Work out the finished part from the listing and answer in its coordinate system (mm). Coordinates: 2 decimals unless noted, no trailing zeros. Order: outer loops, then holes, each group sorted by start corner. A loop starts at its lowest first (then second) coordinate and runs counter-clockwise, first axis right, second up. Notation, with made-up numbers: M 3,7 L 10,7 A22 cw 10,23 Z; hole C 88.5,83 d10. An arc over 180 degrees is marked long. Use a Markdown table: item, result. Add a question column.
from build123d import *

# Parameters (mm, degrees)
SKETCH1_R           = 1.5
BOSS_EXTRUDE1_DEPTH = 40


with BuildPart() as part:
    # Sketch1 → Boss-Extrude1 (new body)
    with BuildSketch(Plane(origin=(0, 0, 0), x_dir=(1, 0, 0), z_dir=(0, 1, 0))):
        Polygon((0, 2.886751346), (-2.5, 1.443375673), (-2.5, -1.443375673), (0, -2.886751346), (2.5, -1.443375673), (2.5, 1.443375673), align=None)
        with Locations(Location((0, 0, 0), (0, 0, 270))):
            Circle(SKETCH1_R, mode=Mode.SUBTRACT)
    extrude(amount=BOSS_EXTRUDE1_DEPTH)

    # Sketch6 → Cut-Revolve1 (revolve, cut)
    with BuildSketch(Plane.ZY):
        Polygon((2.5, 40), (2.886751346, 40), (2.886751346, 39.859234022), align=None)
    cut_revolve1 = revolve(axis=Axis((0, 40, 0), (0, 1, 0)), mode=Mode.SUBTRACT)

    # Mirror1: Cut-Revolve1 across plane
    add(cut_revolve1.mirror(Plane.ZX.offset(20)), mode=Mode.SUBTRACT)


solid = part.part
(1) Given P1, Ø3, axis at x = 1, y = 6.5, coming from the +Z side, flat-ended and moving along its own axis, determine where the tip first touches the part or whether it passes through.
(2) The mould has two halves that part along X. Classify faces 1 (the flat face through (-2.5, 20, 0)), 2 (the conical face through (2.31, 39.94, -1.33)), 3 (the cylindrical face through (0.45, 19.72, 1.43)), 4 (the flat face through (2, 0, 0)): pulls with the +X half, pulls with the -X half, needs draft (parallel to the pull), parting line crosses it, or undercut.
(3) A cutting plane is placed at A-A on y = 10. Write down the section's boundary in (x, z), plus the area to 3 significant figures.
(4) Straight lines are drawn through the part: line 1 (X direction, y = 35, z = 0); line 2 (X direction, y = 5.5, z = -0.4); line 3 (Z direction, x = 0.95, y = 29.5). For each, find the intervals that lie inside material, in ascending order.
From the geometry:
| question | item | result |
|---|---|---|
| 1 | P1 | stops at z = 2.89 |
| 2 | face 1 | pulls with the -X half |
| 2 | face 2 | pulls with the +X half |
| 2 | face 3 | undercut |
| 2 | face 4 | needs draft |
| 3 | outline | M -2.5,-1.44 L 0,-2.89 L 2.5,-1.44 L 2.5,1.44 L 0,2.89 L -2.5,1.44 Z; hole C 0,0 d3 |
| 3 | area | 14.6 mm2 |
| 4 | line 1 | x = -2.5 to -1.5, 1.5 to 2.5 |
| 4 | line 2 | x = -2.5 to -1.45, 1.45 to 2.5 |
| 4 | line 3 | z = -2.34 to -1.16, 1.16 to 2.34 |
